```python
from build123d import *

# Parameters (mm, degrees)
F1_DEPTH = 4.064


with BuildPart() as f1:
    # F0 (on Front) → F1 (new body)
    with BuildSketch(Plane.XZ):
        with BuildLine():
            Line((4.29974, 1.5875), (0, 1.5875))
            Line((0, 1.5875), (-4.29974, 1.5875))
            ThreePointArc((-4.29974, 1.5875), (-8.789868, 2.407738), (-12.7, 4.7625))
            Line((-12.7, 4.7625), (-31.75, 4.7625))
            Line((-31.75, 4.7625), (-31.75, 0))
            Line((-31.75, 0), (-31.75, -4.7625))
            Line((-31.75, -4.7625), (-12.7, -4.7625))
            ThreePointArc((-12.7, -4.7625), (-8.789868, -2.407738), (-4.29974, -1.5875))
            Line((-4.29974, -1.5875), (0, -1.5875))
            Line((0, -1.5875), (4.29974, -1.5875))
            ThreePointArc((4.29974, -1.5875), (8.789868, -2.407738), (12.7, -4.7625))
            Line((12.7, -4.7625), (31.75, -4.7625))
            Line((31.75, -4.7625), (31.75, 0))
            Line((31.75, 0), (31.75, 4.7625))
            Line((31.75, 4.7625), (12.7, 4.7625))
            ThreePointArc((12.7, 4.7625), (8.789868, 2.407738), (4.29974, 1.5875))
        make_face()
    extrude(amount=F1_DEPTH)


solid = f1.part
```
Work out the finished part from the listing and answer in its coordinate system (mm). A direction names the side the tool comes from. Coordinates: 2 decimals unless noted, no trailing zeros. Write each loop counter-clockwise with the first axis right and the second up, starting at its lowest first coordinate (ties: lowest second). Pieces come first, ordered by that corner, then holes. Notation, with made-up numbers: (88, -10) - (130, -10) arc R34 ccw to (130, 20) - close; hole circle Ø7 at (40, 78.5). An arc over 180 degrees is marked (long way). Answer as a JSON object with one key per item and string values.
Q1. For a pull along X with two mould halves and no side action, classify faces 1 (the flat face through (-31.75, -2, 0)), 2 (the cylindrical face through (8.73, -2.004, -2.385)), 3 (the flat face through (0, -4.064, 0)), 4 (the flat face through (31.75, -2, 0)) as pulls with the +X half, pulls with the -X half, needs draft (parallel to the pull), parting line crosses it, or undercut.
Results list:
{"face 1": "pulls with the -X half", "face 2": "undercut", "face 3": "needs draft", "face 4": "pulls with the +X half"}
Q2. Find section B-B (y = -3.5). Write down the section's boundary in (x, z), plus the area to 3 significant figures.
Results list:
{"outline": "(-31.75, -4.76) - (-12.7, -4.76) arc R12.7 cw to (-4.3, -1.59) - (4.3, -1.59) arc R12.7 cw to (12.7, -4.76) - (31.75, -4.76) - (31.75, 4.76) - (12.7, 4.76) arc R12.7 cw to (4.3, 1.59) - (-4.3, 1.59) arc R12.7 cw to (-12.7, 4.76) - (-31.75, 4.76) - close", "area": "477 mm^2"}
Q3. Find section A-A (z = -3.75). Write down the section's boundary in (x, y).
Results list:
{"outline": "(-31.75, -4.06) - (-11.39, -4.06) - (-11.39, 0) - (-31.75, 0) - close; (11.39, -4.06) - (31.75, -4.06) - (31.75, 0) - (11.39, 0) - close"}
Q4. Given pin 1 Ø2 at (x, y) = (1.5, -2.5) entering from +Z, flat-ended and moving along its own axis, determine where the tip first touches the part or whether it passes through.
Results list:
{"pin 1": "stops at z = 1.59"}
Q5. Find section C-C (z = 3.25). Write down the section's boundary in (x, y), plus the area to 3 significant figures.
Results list:
{"outline": "(-31.75, -4.06) - (-10.58, -4.06) - (-10.58, 0) - (-31.75, 0) - close; (10.58, -4.06) - (31.75, -4.06) - (31.75, 0) - (10.58, 0) - close", "area": "172 mm^2"}
Q6. Consider L1, parallel to X at y = -2.1, z = -4; L2, parallel to X at y = -0.8, z = 2.5; L3, parallel to Z at x = -0.5, y = -1.35. Determine where each line is inside the solid, lowest interval first. Write a range as from..to.
Results list:
{"L1": "x = -31.75..-11.75, 11.75..31.75", "L2": "x = -31.75..-9.03, 9.03..31.75", "L3": "z = -1.59..1.59"}
Q7. Find section D-D (x = 0.5). Write down the section's boundary in (y, z), plus the area to 3 significant figures.
Results list:
{"outline": "(-4.06, -1.59) - (0, -1.59) - (0, 1.59) - (-4.06, 1.59) - close", "area": "12.9 mm^2"}
Q8. Which of the six approach directions +Z, -Z, +X, -X, +Y, -Y give full straight-line access (tool end or side, diameter ignored) to faces 5 (the flat face through (0, 0, 0)), 6 (the cylindrical face through (-8.85, -2, -2.43)), 7 (the cylindrical face through (-8.73, -2.004, 2.385))?
Results list:
{"face 5": "+Z, -Z, +X, -X, +Y", "face 6": "-Z, +Y, -Y", "face 7": "+Z, +Y, -Y"}
